Verification items for the finished model (mm, model axes). Coordinates: 2 decimals unless noted, no trailing zeros. Loops run counter-clockwise (first coordinate to the right, second up) from the corner with the lowest first, then second, coordinate; pieces in that order, holes last. Notation, with made-up numbers: (-37.75, 41.5) -> (7.25, 41.5) arc R24 ccw to (7.25, 77.5) -> close; hole circle Ø10 at (33.5, 34.5). An arc over 180 degrees is marked (long way). Write item = value, one per line.
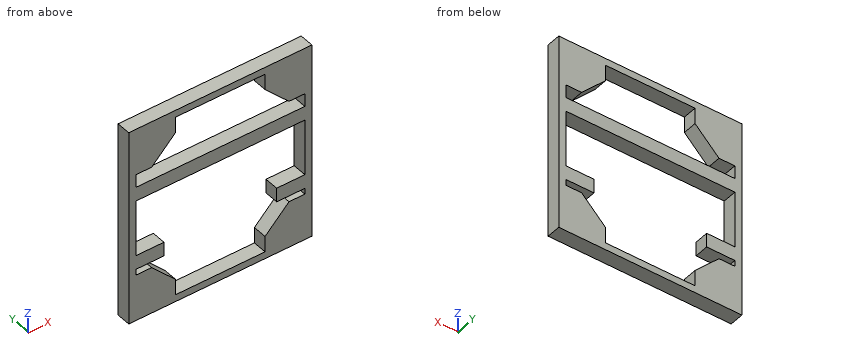
```python
from build123d import *

# Parameters (mm, degrees)
SKETCH1_W           = 660.4
SKETCH1_H           = 711.2
SKETCH1_W_2         = 609.6
SKETCH1_H_2         = 660.4
BOSS_EXTRUDE1_DEPTH = 50.8
SKETCH2_W           = 609.6
SKETCH2_H           = 50.8
BOSS_EXTRUDE2_DEPTH = 50.8
SKETCH3_W           = 406.4
SKETCH3_H           = 50.8
CUT_EXTRUDE2_DEPTH  = 972.861224661


with BuildPart() as part:
    # Sketch1 → Boss-Extrude1 (new body)
    # profile 1 of 5: a face of its own
    with BuildSketch(Plane(origin=(0, 0, 0), x_dir=(1, 0, 0), z_dir=(0, 1, 0))):
        with Locations((330.2, 355.6)):
            Rectangle(SKETCH1_W, SKETCH1_H)
        with Locations((330.2, 355.6)):
            Rectangle(SKETCH1_W_2, SKETCH1_H_2, mode=Mode.SUBTRACT)
    # profile 2 of 5: a face of its own
    with BuildSketch(Plane(origin=(0, 0, 0), x_dir=(1, 0, 0), z_dir=(0, 1, 0))):
        Polygon((82.55, 168.89717139), (25.4, 168.89717139), (25.4, 25.4), (168.89717139, 25.4), (168.89717139, 82.55), align=None)
    # profile 3 of 5: a face of its own
    with BuildSketch(Plane(origin=(0, 0, 0), x_dir=(1, 0, 0), z_dir=(0, 1, 0))):
        Polygon((491.50282861, 82.55), (491.50282861, 25.4), (635, 25.4), (635, 168.89717139), (577.85, 168.89717139), align=None)
    # profile 4 of 5: a face of its own
    with BuildSketch(Plane(origin=(0, 0, 0), x_dir=(1, 0, 0), z_dir=(0, 1, 0))):
        Polygon((635, 685.8), (491.50282861, 685.8), (491.50282861, 628.65), (577.85, 542.30282861), (635, 542.30282861), align=None)
    # profile 5 of 5: a face of its own
    with BuildSketch(Plane(origin=(0, 0, 0), x_dir=(1, 0, 0), z_dir=(0, 1, 0))):
        Polygon((25.4, 542.30282861), (82.55, 542.30282861), (168.89717139, 628.65), (168.89717139, 685.8), (25.4, 685.8), align=None)
    extrude(amount=BOSS_EXTRUDE1_DEPTH)

    # Sketch2 → Boss-Extrude2 (add)
    with BuildSketch(Plane(origin=(0, 50.8, 0), x_dir=(1, 0, 0), z_dir=(0, 1, 0))):
        with Locations((330.2, 241.3)):
            Rectangle(SKETCH2_W, SKETCH2_H)
        with Locations((330.2, 495.3)):
            Rectangle(SKETCH2_W, SKETCH2_H)
    extrude(amount=-BOSS_EXTRUDE2_DEPTH)

    # Sketch3 → Cut-Extrude2 (cut, through all)
    with BuildSketch(Plane(origin=(0, 50.8, 0), x_dir=(1, 0, 0), z_dir=(0, 1, 0))):
        with Locations((330.2, 495.3)):
            Rectangle(SKETCH3_W, SKETCH3_H)
    extrude(amount=-CUT_EXTRUDE2_DEPTH, mode=Mode.SUBTRACT)


solid = part.part
```
1) Sectioned sample at C-C, the plane y = 41.5. Count the separate pieces of the cut face and the enclosed holes in it, plus the area to 3 significant figures.
Ans:
separate_pieces = 1
enclosed_holes = 2
area = 176,000 mm2
2) Sectioned sample at A-A, the plane x = 601. Record the cut outline in (y, z).
Ans:
outline = (0, -711.2) -> (50.8, -711.2) -> (50.8, -542.3) -> (0, -542.3) -> close; (0, -520.7) -> (50.8, -520.7) -> (50.8, -469.9) -> (0, -469.9) -> close; (0, -266.7) -> (50.8, -266.7) -> (50.8, -215.9) -> (0, -215.9) -> close; (0, -168.9) -> (50.8, -168.9) -> (50.8, 0) -> (0, 0) -> close
3) Sectioned sample at D-D, the plane x = 370.5. Record the cut outline in (y, z).
Ans:
outline = (0, -711.2) -> (50.8, -711.2) -> (50.8, -685.8) -> (0, -685.8) -> close; (0, -266.7) -> (50.8, -266.7) -> (50.8, -215.9) -> (0, -215.9) -> close; (0, -25.4) -> (50.8, -25.4) -> (50.8, 0) -> (0, 0) -> close
4) Material ranges on line 1 (Z direction, x = 388.5, y = 6); line 2 (Z direction, x = 631.5, y = 25); line 3 (X direction, y = 25, z = -450), recorded low to high.
Ans:
line_1 = -711.2 to -685.8, -266.7 to -215.9, -25.4 to 0
line_2 = -711.2 to -542.3, -520.7 to -469.9, -266.7 to -215.9, -168.9 to 0
line_3 = 0 to 25.4, 635 to 660.4
5) Sectioned sample at B-B, the plane z = -403. Record the cut outline in (x, y), plus the area to 3 significant figures.
Ans:
outline = (0, 0) -> (25.4, 0) -> (25.4, 50.8) -> (0, 50.8) -> close; (635, 0) -> (660.4, 0) -> (660.4, 50.8) -> (635, 50.8) -> close
area = 2,580 mm2
